from build123d import *

# Parameters (mm, degrees)
BOSS_EXTRUDE1_DEPTH = 3.175
SKETCH3_R           = 2.032
CUT_EXTRUDE1_DEPTH  = 385.384860036
FILLET1_R           = 1.5875


with BuildPart() as part:
    # Sketch2 → Boss-Extrude1 (new body)
    with BuildSketch(Plane(origin=(0, 0, 0), x_dir=(1, 0, 0), z_dir=(0, 1, 0))):
        with BuildLine():
            Line((0, 7.00756403), (0, 50.8))
            Line((0, 50.8), (381, 50.8))
            Line((381, 50.8), (381, 7.00756403))
            ThreePointArc((381, 7.00756403), (380.879158758, 6.400054081), (380.535032015, 5.885032015))
            Line((380.535032015, 5.885032015), (375.114967985, 0.464967985))
            ThreePointArc((375.114967985, 0.464967985), (374.599945919, 0.120841242), (373.99243597, 0))
            Line((373.99243597, 0), (7.00756403, 0))
            ThreePointArc((7.00756403, 0), (6.400054081, 0.120841242), (5.885032015, 0.464967985))
            Line((5.885032015, 0.464967985), (0.464967985, 5.885032015))
            ThreePointArc((0.464967985, 5.885032015), (0.120841242, 6.400054081), (0, 7.00756403))
        make_face()
    extrude(amount=BOSS_EXTRUDE1_DEPTH)

    # Sketch3 → Cut-Extrude1 (cut, through all)
    with BuildSketch(Plane(origin=(0, 0, 0), x_dir=(1, 0, 0), z_dir=(0, 1, 0))):
        with Locations(Location((4.7625, 7.9375, 0), (0, 0, 270))):
            Circle(SKETCH3_R)
        with Locations(Location((4.7625, 46.0375, 0), (0, 0, 270))):
            Circle(SKETCH3_R)
        with Locations(Location((376.2375, 7.9375, 0), (0, 0, 270))):
            Circle(SKETCH3_R)
        with Locations(Location((376.2375, 46.0375, 0), (0, 0, 270))):
            Circle(SKETCH3_R)
        with Locations(Location((341.884, 25.4, 0), (0, 0, 270))):
            Circle(SKETCH3_R)
        with Locations(Location((247.65, 44.45, 0), (0, 0, 270))):
            Circle(SKETCH3_R)
        with Locations(Location((284.734, 44.45, 0), (0, 0, 270))):
            Circle(SKETCH3_R)
        with Locations(Location((247.65, 6.35, 0), (0, 0, 270))):
            Circle(SKETCH3_R)
        with Locations(Location((284.734, 6.35, 0), (0, 0, 270))):
            Circle(SKETCH3_R)
        with Locations(Location((190.5, 25.4, 0), (0, 0, 270))):
            Circle(SKETCH3_R)
        with Locations(Location((133.35, 44.45, 0), (0, 0, 270))):
            Circle(SKETCH3_R)
        with Locations(Location((96.266, 44.45, 0), (0, 0, 270))):
            Circle(SKETCH3_R)
        with Locations(Location((96.266, 6.35, 0), (0, 0, 270))):
            Circle(SKETCH3_R)
        with Locations(Location((77.724, 25.4, 0), (0, 0, 270))):
            Circle(SKETCH3_R)
        with Locations(Location((39.116, 25.4, 0), (0, 0, 270))):
            Circle(SKETCH3_R)
        with Locations(Location((151.892, 25.4, 0), (0, 0, 270))):
            Circle(SKETCH3_R)
        with Locations(Location((229.108, 25.4, 0), (0, 0, 270))):
            Circle(SKETCH3_R)
        with Locations(Location((266.192, 25.4, 0), (0, 0, 270))):
            Circle(SKETCH3_R)
        with Locations(Location((303.276, 25.4, 0), (0, 0, 270))):
            Circle(SKETCH3_R)
        with Locations(Location((114.808, 25.4, 0), (0, 0, 270))):
            Circle(SKETCH3_R)
    extrude(amount=CUT_EXTRUDE1_DEPTH, mode=Mode.SUBTRACT)

    # Fillet1
    fillet1_edges = [part.edges().sort_by_distance(p)[0] for p in [
        (381, 1.5875, -50.8),
        (0, 1.5875, -50.8),
    ]]
    fillet(fillet1_edges, radius=FILLET1_R)


solid = part.part
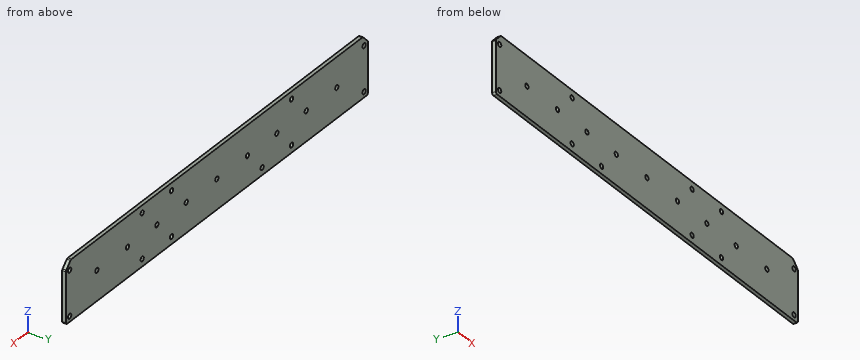
Source: CAD feature listing. Evaluate the final solid. Frame: model axes, mm. Give positions to 0.01 mm unless a question says otherwise; leave off trailing zeros. Write item = value, one per line.
Q1. Cut plane A-A, the plane y = 1.05. State how many separate pieces and enclosed holes the cut face has, and give its area (3 significant figures).
Data:
separate_pieces = 1
enclosed_holes = 20
area = 19,100 mm^2
Q2. Material intervals for line 1 (Z direction, x = 133, y = 2.45); line 2 (X direction, y = 0.5, z = -7); line 3 (X direction, y = 3, z = -4), sorted ascending. Write a range as from..to.
Data:
line_1 = -50.8..-46.45, -42.45..0
line_2 = 0..2.96, 6.57..94.34, 98.19..245.72, 249.58..282.81, 286.66..374.43, 378.04..381
line_3 = 2.35..378.65
Q3. Pin query (flat end, axial travel): pin 1 (6.5 mm diameter, centred on x = 266.192, z = -25.4, fed in from -Y). Return the tip coordinate at first contact, or that it passes through.
Data:
pin_1 = 0
